The figure shows three views and two pictorial views of one solid part (mm, origin at its lowest corner). Answer the questions. A direction names the side the tool comes from. Give positions to 0.01 mm unless a question says otherwise; leave off trailing zeros. Order: outer loops, then holes, each group sorted by start corner. A loop starts at its lowest first (then second) coordinate and runs counter-clockwise, first axis right, second up. Notation, with made-up numbers: (86.25, 4.5) - (104.25, 4.5) arc R22 cw to (104.25, 16.5) - close; hole circle Ø10 at (29, 47.5). An arc over 180 degrees is marked (long way). Answer as a JSON object with one key per item and string values. Group by question number.
Q1. Given pin 1 (0.8 mm diameter, centred on x = 1.5, z = 1, fed in from +Y); pin 2 (0.9 mm diameter, centred on x = 1.5, y = 2.5, fed in from -Z); pin 3 (1 mm diameter, centred on y = 3, z = 4.5, fed in from +X), each flat-ended and moving along its own axis, determine where each tip first touches the part or whether it passes through.
Q2. A cutting plane is placed at A-A, the plane x = 2. Give the vertices of the cut face in (y, z).
Q3. A cutting plane is placed at B-B, the plane z = 6.5. Give the vertices of the cut face in (x, y).
Q4. For the marked faces 4 and 5, determine the directions among +Z, -Z, +X, -X, +Y, -Y from which every point of the face is accessible in a straight line to the end or side of a thin tool.
Q5. The mould has two halves that part along Y. Classify the marked faces 1, 2 and 3: released by +Y, released by -Y, zero draft, split by the parting line, or undercut.
Q6. Consider line 1 (Y direction, x = 1.1, z = 1); line 2 (Y direction, x = 2.05, z = 4.5); line 3 (Z direction, x = 3.4, y = 1.15). Determine where each line is inside the solid, lowest interval first.
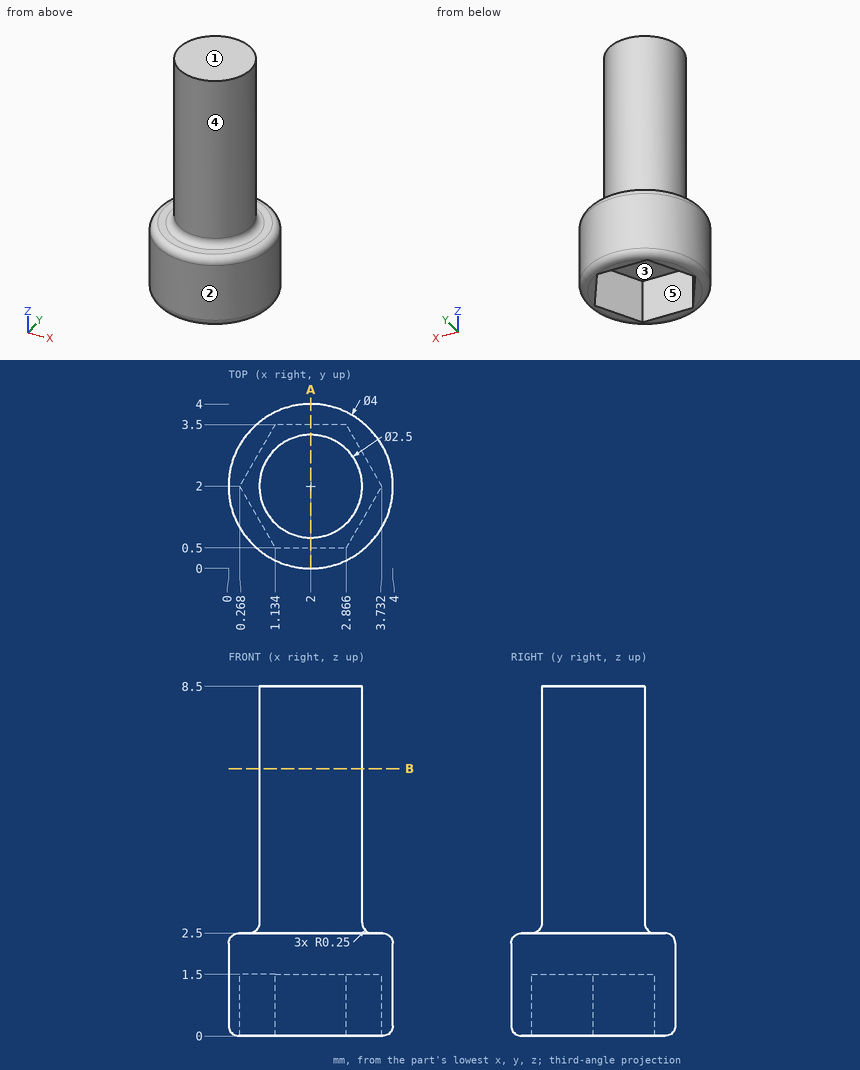
Reply:
{
 "1": {"pin 1": "stops at y = 4", "pin 2": "stops at z = 1.5", "pin 3": "stops at x = 3.15"},
 "2": {"outline": "(0, 0.25) arc R0.25 ccw to (0.25, 0) - (0.5, 0) - (0.5, 1.5) - (3.5, 1.5) - (3.5, 0) - (3.75, 0) arc R0.25 ccw to (4, 0.25) - (4, 2.25) arc R0.25 ccw to (3.75, 2.5) - (3.5, 2.5) arc R0.25 cw to (3.25, 2.75) - (3.25, 8.5) - (0.75, 8.5) - (0.75, 2.75) arc R0.25 cw to (0.5, 2.5) - (0.25, 2.5) arc R0.25 ccw to (0, 2.25) - close"},
 "3": {"outline": "circle Ø2.5 at (2, 2)"},
 "4": {"face 4": "+Z", "face 5": "-Z"},
 "5": {"face 1": "zero draft", "face 2": "split by the parting line", "face 3": "undercut"},
 "6": {"line 1": "y = 0.21 to 0.56, 3.44 to 3.79", "line 2": "y = 0.75 to 3.25", "line 3": "z = 0 to 2.5"}
}
